Work out the finished part from the listing and answer in its coordinate system (mm). A direction names the side the tool comes from. Round coordinates to 2 decimals unless told otherwise and drop trailing zeros. Loops run counter-clockwise (first coordinate to the right, second up) from the corner with the lowest first, then second, coordinate; pieces in that order, holes last. Notation, with made-up numbers: (73.25, -21.75) - (130.25, -21.75) arc R24 ccw to (130.25, 17.25) - close; hole circle Ø8 at (66.5, 25). An arc over 180 degrees is marked (long way). Use CSV: the item, a comma, the result in double quotes. Start each with the question number.
from build123d import *

# Parameters (mm, degrees)
F0_R     = 50
F1_DEPTH = 2
F2_R     = 50
F2_R_2   = 45
F3_DEPTH = 5
F3_TAPER = 5
F5_DEPTH = 5


with BuildPart() as f1:
    # F0 (on Top) → F1 (new body)
    with BuildSketch(Plane.XY):
        Circle(F0_R)
    extrude(amount=F1_DEPTH)

    # F2 (on face) → F3 (join)
    with BuildSketch(Plane.XY.offset(2)):
        Circle(F2_R)
        Circle(F2_R_2, mode=Mode.SUBTRACT)
    extrude(amount=F3_DEPTH, taper=F3_TAPER)

    # F4 (on face) → F5 (join, through all)
    with BuildSketch(Plane.XY.offset(2)):
        Polygon((-18, -25), (0, -25), (18, -25), (18, 15), (0, 33), (-18, 15), align=None)
    extrude(amount=F5_DEPTH)


solid = f1.part
Item 1: Each of these flat-tipped pins is pushed along its axis until it touches: pin 1 Ø3 at (y, z) = (10, 3) entering from -X; pin 2 Ø4 at (y, z) = (27, 6) entering from -X; pin 3 Ø3 at (x, z) = (-6.5, 2) entering from +Y. Where does it stop, or does it pass through?
Item 2: Find the intervals of material crossed by probe 1 along X at (y, z) = (-17, 3.5); probe 2 along X at (y, z) = (16, 5.5); probe 3 along Y at (x, z) = (11.5, 3), in increasing order. Write a range as [from, to].
Item 3: A cutting plane is placed at A-A (z = 5.5). Determine the outline of the cut face in (x, y), plus the area to 3 significant figures.
Item 4: The mould has two halves that part along Y. Classify faces 3 (the flat face through (0, -2, 7)), 4 (the conical face through (47.294, 14.894, 6.757)), 5 (the flat face through (19, 1, 2)): pulls with the +Y half, pulls with the -Y half, needs draft (parallel to the pull), parting line crosses it, or undercut.
Item 5: Which of the six approach directions +Z, -Z, +X, -X, +Y, -Y give full straight-line access (tool end or side, diameter ignored) to faces 1 (the flat face through (-1, 1, 0)), 2 (the flat face through (0, -25, 4))?
Result sheet:
1,pin 1,"x = -49.22"
1,pin 2,"x = -42.91"
1,pin 3,"y = 49.75"
2,probe 1,"[-46.88, -41.81], [-18, 18], [41.81, 46.88]"
2,probe 2,"[-47.05, -42.39], [-17, 17], [42.39, 47.05]"
2,probe 3,"[-48.57, -43.6], [-25, 21.5], [43.6, 48.57]"
3,outline,"circle Ø99.39 at (0, 0); (-18, -25) - (18, -25) - (18, 15) - (0, 33) - (-18, 15) - close; hole circle Ø90.61 at (0, 0)"
3,area,"3,070 mm^2"
4,face 3,"needs draft"
4,face 4,"parting line crosses it"
4,face 5,"undercut"
5,face 1,"-Z, +X, -X, +Y, -Y"
5,face 2,"+Z"
